```python
from build123d import *

# Parameters (mm, degrees)
F0_W          = 1
F0_H          = 1.375
F1_DEPTH      = 16
F0_W_2        = 0.65
F0_H_2        = 0.65
F2_DEPTH      = 1.25
F3_W          = 2.15
F3_H          = 2.65
F4_DEPTH      = 1.2
F5_R          = 1
F6_W          = 8.9
F6_H          = 5.9
F7_DEPTH      = 0.5
F7_TAPER      = 3
F8_DEPTH      = 7
F8_DEPTH_BACK = 0.9
F9_SIZE       = 0.3


# Not quite as in the source:
# - a feature names something its author has since deleted; it is built from what else it names


with BuildPart() as f1:
    # F0 (on Front) → F1 (new body)
    with BuildSketch(Plane.XZ):
        Polygon((-1.15, 11.35), (-1.15, -1.15), (-0.45, -1.15), (-0.45, -2.775), (0.55, -2.775), (0.55, -1.15), (14.3, -1.15), (14.3, 2.675), (15.2, 2.675), (15.2, 7.525), (14.3, 7.525), (14.3, 11.35), (9.2, 11.35), (9.2, 12.975), (8.2, 12.975), (8.2, 11.35), align=None)
        Polygon((13.2, 0), (0, 0), (0, 10), (11, 10), (11, 8.325), (13.2, 8.325), (13.2, 7.425), (11, 7.425), (11, 6.425), (14, 6.425), (14, 3.775), (11, 3.775), (11, 0.9), (13.2, 0.9), align=None, mode=Mode.SUBTRACT)
        with Locations((8.7, 13.6625)):
            Rectangle(F0_W, F0_H)
        with Locations((0.05, -3.4625)):
            Rectangle(F0_W, F0_H)
    extrude(amount=-F1_DEPTH)

    # F0 (on Front) → F2 (join)
    with BuildSketch(Plane.XZ):
        Polygon((-1.15, 11.35), (-1.15, -1.15), (-0.45, -1.15), (-0.45, -2.775), (0.55, -2.775), (0.55, -1.15), (14.3, -1.15), (14.3, 2.675), (15.2, 2.675), (15.2, 7.525), (14.3, 7.525), (14.3, 11.35), (9.2, 11.35), (9.2, 12.975), (8.2, 12.975), (8.2, 11.35), align=None)
        Polygon((13.2, 0), (0, 0), (0, 10), (11, 10), (11, 8.325), (13.2, 8.325), (13.2, 7.425), (11, 7.425), (11, 6.425), (14, 6.425), (14, 3.775), (11, 3.775), (11, 0.9), (13.2, 0.9), align=None, mode=Mode.SUBTRACT)
        Polygon((-0.45, -1.15), (-1.15, -1.15), (-1.15, 11.35), (8.2, 11.35), (8.2, 12.975), (-6.2, 12.975), (-6.2, -2.775), (-0.45, -2.775), align=None)
        with Locations((0.05, -3.4625)):
            Rectangle(F0_W, F0_H)
        Polygon((0.55, -1.15), (0.55, -2.775), (16.45, -2.775), (16.45, 12.975), (9.2, 12.975), (9.2, 11.35), (14.3, 11.35), (14.3, 7.525), (15.2, 7.525), (15.2, 2.675), (14.3, 2.675), (14.3, -1.15), align=None)
        with Locations((8.7, 13.6625)):
            Rectangle(F0_W, F0_H)
        Polygon((0, 10), (0, 0), (13.2, 0), (13.2, 0.9), (11, 0.9), (11, 3.775), (14, 3.775), (14, 6.425), (11, 6.425), (11, 7.425), (13.2, 7.425), (13.2, 8.325), (11, 8.325), (11, 10), align=None)
        with Locations((2.96, 3.83)):
            Rectangle(F0_W_2, F0_H_2, mode=Mode.SUBTRACT)
        with Locations((5.5, 3.83)):
            Rectangle(F0_W_2, F0_H_2, mode=Mode.SUBTRACT)
        with Locations((8.04, 3.83)):
            Rectangle(F0_W_2, F0_H_2, mode=Mode.SUBTRACT)
        with Locations((2.96, 6.37)):
            Rectangle(F0_W_2, F0_H_2, mode=Mode.SUBTRACT)
        with Locations((5.5, 6.37)):
            Rectangle(F0_W_2, F0_H_2, mode=Mode.SUBTRACT)
        with Locations((8.04, 6.37)):
            Rectangle(F0_W_2, F0_H_2, mode=Mode.SUBTRACT)
    extrude(amount=F2_DEPTH)

    # F3 (on face) → F4 (cut, through all)
    with BuildSketch(Plane.YZ.offset(15.2)):
        with Locations((11.925, 5.1)):
            Rectangle(F3_W, F3_H)
    extrude(amount=-F4_DEPTH, mode=Mode.SUBTRACT)

    # F5
    f5_edges = [f1.edges().sort_by_distance(p)[0] for p in [
        (16.45, -0.625, 12.975),
        (-6.2, -0.625, 12.975),
        (16.45, -0.625, -2.775),
        (-6.2, -0.625, -2.775),
    ]]
    fillet(f5_edges, radius=F5_R)

    # F6 (on face) → F7 (cut)
    with BuildSketch(Plane.XZ.offset(1.25)):
        with Locations((5.25, 5.1)):
            Rectangle(F6_W, F6_H)
    extrude(amount=-F7_DEPTH, taper=F7_TAPER, mode=Mode.SUBTRACT)

    # F0 (on Front) → F8 (join, two sides)
    with BuildSketch(Plane.XZ) as f8_sk:
        with Locations((2.96, 6.37)):
            Rectangle(F0_W_2, F0_H_2)
        with Locations((5.5, 6.37)):
            Rectangle(F0_W_2, F0_H_2)
        with Locations((8.04, 6.37)):
            Rectangle(F0_W_2, F0_H_2)
        with Locations((2.96, 3.83)):
            Rectangle(F0_W_2, F0_H_2)
        with Locations((5.5, 3.83)):
            Rectangle(F0_W_2, F0_H_2)
        with Locations((8.04, 3.83)):
            Rectangle(F0_W_2, F0_H_2)
    extrude(amount=-F8_DEPTH)
    extrude(f8_sk.sketch, amount=F8_DEPTH_BACK)

    # F9
    f9_edges = [f1.edges().sort_by_distance(p)[0] for p in [
        (12.1, 16, 7.425),
        (13.2, 16, 7.875),
        (5.5, 16, 10),
        (0, 16, 5),
        (6.6, 16, 0),
        (12.1, 16, 0.9),
        (13.2, 16, 0.45),
        (11, 16, 2.3375),
        (12.5, 16, 3.775),
        (14, 16, 5.1),
        (12.5, 16, 6.425),
        (11, 16, 6.925),
        (12.1, 16, 8.325),
        (11, 16, 9.1625),
    ]]
    chamfer(f9_edges, length=F9_SIZE)


solid = f1.part
```
The listing builds one solid part. Answer for the finished solid, in the listing's coordinates (mm). A direction names the side the tool comes from. Coordinates: 2 decimals unless noted, no trailing zeros. Loops run counter-clockwise (first coordinate to the right, second up) from the corner with the lowest first, then second, coordinate; pieces in that order, holes last. Notation, with made-up numbers: (68, -13) -> (99, -13) arc R22 cw to (99, -7) -> close; hole circle Ø11 at (-18, 1.5). An arc over 180 degrees is marked (long way). Return JSON: item names as keys, results as strings. Group by question number.
(1) A cutting plane is placed at C-C on z = 0.5. Write down the section's boundary in (x, y).
(2) Determine the mould class of faces 1 (the flat face through (13, 8, 6.425)), 2 (the flat face through (-1.15, 8, 5)), 3 (the flat face through (15, 8, 2.675)), 4 (the flat face through (12, 8, 11.35)) for opening direction Z: released by +Z, released by -Z, zero draft, split by the parting line, or undercut.
(3) Given pin 1 Ø4 at (y, z) = (6.5, 0) entering from +X; pin 2 Ø0.7 at (x, z) = (8, 4) entering from -Y; pin 3 Ø1 at (x, y) = (1, 11.5) entering from +Z, each flat-ended and moving along its own axis, determine where each tip first touches the part or whether it passes through.
(4) A cutting plane is placed at D-D on y = 4. Count the separate pieces of the cut face and the enclosed holes in it, and give its area (3 significant figures).
(5) Which of the six approach directions +Z, -Z, +X, -X, +Y, -Y give full straight-line access (tool end or side, diameter ignored) to faces 5 (the flat face through (14.3, 8, 1)), 6 (the flat face through (4, 8, 11.35)), 7 (the flat face through (15.2, 8, 5)), 8 (the flat face through (12, 8, 7.425))?
(6) Find the intervals of material crossed by probe 1 along Z at (x, y) = (5.25, 5.75) (3 decimals); probe 2 along Z at (x, y) = (12.25, 13.25) (3 decimals); probe 3 along X at (y, z) = (2.5, 2.5), in increasing order. Write a range as from..to.
(7) A cutting plane is placed at B-B on x = 10. Write down the section's boundary in (y, z) (3 decimals).
The answers:
{
 "1": {"outline": "(-6.2, -1.25) -> (16.45, -1.25) -> (16.45, 0) -> (14.3, 0) -> (14.3, 16) -> (13.5, 16) -> (13.2, 15.7) -> (13.2, 0) -> (0, 0) -> (0, 15.7) -> (-0.3, 16) -> (-1.15, 16) -> (-1.15, 0) -> (-6.2, 0) -> close"},
 "2": {"face 1": "undercut", "face 2": "zero draft", "face 3": "released by -Z", "face 4": "released by +Z"},
 "3": {"pin 1": "stops at x = 14.3", "pin 2": "stops at y = -0.9", "pin 3": "stops at z = 11.35"},
 "4": {"separate pieces": "7", "enclosed holes": "1", "area": "84.1 mm^2"},
 "5": {"face 5": "-Z, +X, +Y", "face 6": "+Z, -X, +Y", "face 7": "+Z, -Z, +X, +Y", "face 8": "+Y"},
 "6": {"probe 1": "z = -1.15..0, 3.505..4.155, 6.045..6.695, 10..11.35", "probe 2": "z = -1.15..0, 0.9..3.775, 6.425..7.425, 8.325..11.35", "probe 3": "x = -1.15..0, 11..14.3"},
 "7": {"outline": "(-1.25, -2.775) -> (0, -2.775) -> (0, -1.15) -> (16, -1.15) -> (16, -0.3) -> (15.7, 0) -> (0, 0) -> (0, 10) -> (15.7, 10) -> (16, 10.3) -> (16, 11.35) -> (0, 11.35) -> (0, 12.975) -> (-1.25, 12.975) -> close"}
}
